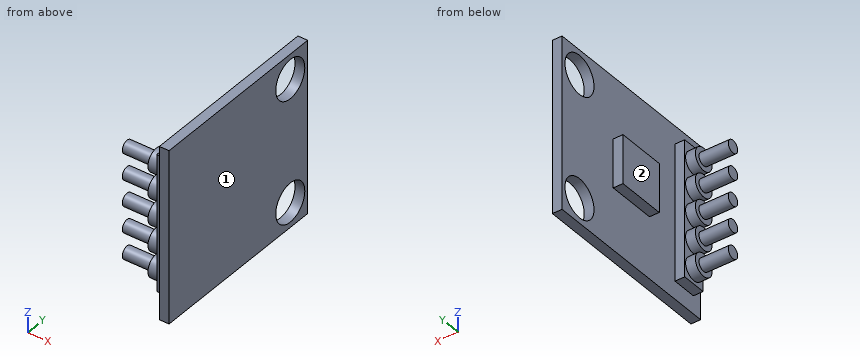
from build123d import *

# Parameters (mm, degrees)
SKETCH1_W           = 17.7
SKETCH1_H           = 19.1
SKETCH1_R           = 2
BOSS_EXTRUDE1_DEPTH = 1
SKETCH2_W           = 14
SKETCH2_H           = 2.54
SKETCH2_W_2         = 5
SKETCH2_H_2         = 5
BOSS_EXTRUDE2_DEPTH = 1
SKETCH3_R           = 1.15
BOSS_EXTRUDE3_DEPTH = 1
SKETCH4_R           = 0.65
BOSS_EXTRUDE4_DEPTH = 3


with BuildPart() as part:
    # Sketch1 → Boss-Extrude1 (new body)
    with BuildSketch(Plane(origin=(0, 0, 0), x_dir=(0, 0, -1), z_dir=(1, 0, 0))):
        with Locations((8.85, 9.55)):
            Rectangle(SKETCH1_W, SKETCH1_H)
        with Locations((15.15, 16.7)):
            Circle(SKETCH1_R, mode=Mode.SUBTRACT)
        with Locations((2.55, 16.7)):
            Circle(SKETCH1_R, mode=Mode.SUBTRACT)
    extrude(amount=BOSS_EXTRUDE1_DEPTH)

    # Sketch2 → Boss-Extrude2 (add)
    with BuildSketch(Plane.ZY):
        with Locations((-8.85, 2.27)):
            Rectangle(SKETCH2_W, SKETCH2_H)
        with Locations((-8.85, 9.55)):
            Rectangle(SKETCH2_W_2, SKETCH2_H_2)
    extrude(amount=BOSS_EXTRUDE2_DEPTH)

    # Sketch3 → Boss-Extrude3 (add)
    with BuildSketch(Plane.ZY.offset(1)):
        with Locations((-14.35, 2.27)):
            Circle(SKETCH3_R)
        with Locations((-11.65, 2.27)):
            Circle(SKETCH3_R)
        with Locations((-8.95, 2.27)):
            Circle(SKETCH3_R)
        with Locations((-6.25, 2.27)):
            Circle(SKETCH3_R)
        with Locations((-3.55, 2.27)):
            Circle(SKETCH3_R)
    extrude(amount=BOSS_EXTRUDE3_DEPTH)

    # Sketch4 → Boss-Extrude4 (add)
    with BuildSketch(Plane.ZY.offset(2)):
        with Locations((-14.35, 2.27)):
            Circle(SKETCH4_R)
        with Locations((-11.65, 2.27)):
            Circle(SKETCH4_R)
        with Locations((-8.95, 2.27)):
            Circle(SKETCH4_R)
        with Locations((-6.25, 2.27)):
            Circle(SKETCH4_R)
        with Locations((-3.55, 2.27)):
            Circle(SKETCH4_R)
    extrude(amount=BOSS_EXTRUDE4_DEPTH)


solid = part.part
Geometry: final body of the model. Coordinates: model frame, mm. Face numbers are marked on the shaded views. A direction names the side the tool comes from. Give positions to 0.01 mm unless a question says otherwise; leave off trailing zeros. Order: outer loops, then holes, each group sorted by start corner. A loop starts at its lowest first (then second) coordinate and runs counter-clockwise, first axis right, second up. Notation, with made-up numbers: (-3.75, 11.25) - (23.25, 11.25) arc R37 ccw to (23.25, 49.25) - close; hole circle Ø11 at (8.25, 59). An arc over 180 degrees is marked (long way). Use CSV: the item, a comma, the result in double quotes.
1. Contact query for flat-ended pins moving along their axis: pin 1 (0.8 mm diameter, centred on x = -0.5, z = -7.5, fed in from -Y); pin 2 (1 mm diameter, centred on x = -1, y = 12.5, fed in from +Z); pin 3 (3 mm diameter, centred on y = 16.7, z = -15.15, fed in from +X); pin 4 (5.5 mm diameter, centred on y = 12.5, z = -6.5, fed in from -X). Output: stop coordinate, or through.
Answers below:
pin 1,"y = 1"
pin 2,"z = -6.35"
pin 3,"through"
pin 4,"x = -1"
2. Material intervals for line 1 along Y through (x, z) = (0.2, -15.15); line 2 along X through (y, z) = (10.5, -7.25); line 3 along X through (y, z) = (8.75, -15), sorted ascending. Write a range as from..to.
Answers below:
line 1,"0..14.7, 18.7..19.1"
line 2,"-1..1"
line 3,"0..1"
3. Section query D-D (y = 11.5). Output: boundary loops of the cut face in (x, z).
Answers below:
outline,"(-1, -11.35) - (0, -11.35) - (0, -17.7) - (1, -17.7) - (1, 0) - (0, 0) - (0, -6.35) - (-1, -6.35) - close"
4. Section query C-C (x = -4.1). Output: boundary loops of the cut face in (y, z), plus the area to 3 significant figures.
Answers below:
outline,"circle Ø1.3 at (2.27, -14.35); circle Ø1.3 at (2.27, -11.65); circle Ø1.3 at (2.27, -8.95); circle Ø1.3 at (2.27, -6.25); circle Ø1.3 at (2.27, -3.55)"
area,"6.64 mm2"
5. Section query A-A (y = 16.7). Output: boundary loops of the cut face in (x, z).
Answers below:
outline,"(0, -17.7) - (1, -17.7) - (1, -17.15) - (0, -17.15) - close; (0, -13.15) - (1, -13.15) - (1, -4.55) - (0, -4.55) - close; (0, -0.55) - (1, -0.55) - (1, 0) - (0, 0) - close"
6. Access query for the marked faces 1 and 2. Directions: +Z, -Z, +X, -X, +Y, -Y. A direction counts if a zero-diameter tool reaches every point of the face in a straight line with its end or side. Return the directions, or none.
Answers below:
face 1,"+Z, -Z, +X, +Y, -Y"
face 2,"+Z, -Z, -X, +Y"
7. Section query B-B (z = -14). Output: boundary loops of the cut face in (x, y).
Answers below:
outline,"(-5, 1.72) - (-2, 1.72) - (-2, 1.17) - (-1, 1.17) - (-1, 1) - (0, 1) - (0, 0) - (1, 0) - (1, 15.06) - (0, 15.06) - (0, 3.54) - (-1, 3.54) - (-1, 3.37) - (-2, 3.37) - (-2, 2.82) - (-5, 2.82) - close; (0, 18.34) - (1, 18.34) - (1, 19.1) - (0, 19.1) - close"
